Part model, mm, in its own coordinate system. A direction names the side the tool comes from. Coordinates: 2 decimals unless noted, no trailing zeros. Loops run counter-clockwise (first coordinate to the right, second up) from the corner with the lowest first, then second, coordinate; pieces in that order, holes last. Notation, with made-up numbers: M 54,9.5 L 93,9.5 A31 cw 93,44.5 Z; hole C -23,56 d6. An arc over 180 degrees is marked long. Use CSV: the item, a comma, the result in double quotes. Start each with the question number.
from build123d import *

# Parameters (mm, degrees)
F0_R     = 3.175
F1_DEPTH = 25.4
F2_R     = 12.7
F3_R     = 12.69999


# Not quite as in the source:
# - a fillet or chamfer is up to 0.001 mm smaller than in the source, because OpenCascade refuses the exact size


with BuildPart() as f1:
    # F0 (on Front) → F1 (new body)
    with BuildSketch(Plane.XZ):
        with BuildLine():
            Line((0, 44.897188701), (0, -74.9478926185))
            Line((0, -74.9478926185), (25.4, -74.9478926185))
            Line((25.4, -74.9478926185), (25.4, 44.897188701))
            ThreePointArc((25.4, 44.897188701), (-28.9774724535, 99.2746611545), (-83.3549449071, 44.897188701))
            Line((-83.3549449071, 44.897188701), (-57.9549449071, 44.897188701))
            ThreePointArc((-57.9549449071, 44.897188701), (-28.9774724535, 73.8746611545), (0, 44.897188701))
        make_face()
        with Locations((12.7, -62.2478926185)):
            Circle(F0_R, mode=Mode.SUBTRACT)
    extrude(amount=F1_DEPTH)

    # F2
    f2_edges = [f1.edges().sort_by_distance(p)[0] for p in [
        (-70.654945, -25.4, 44.897189),
    ]]
    fillet(f2_edges, radius=F2_R)

    # F3 (radius 12.7 in the source; OpenCascade refuses exactly that, so slightly less here)
    f3_edges = [f1.edges().sort_by_distance(p)[0] for p in [
        (-70.654945, 0, 44.897189),
    ]]
    fillet(f3_edges, radius=F3_R)


solid = f1.part
1. Wall check: probe 1 along X at (y, z) = (-9, 15); probe 2 along Z at (x, y) = (15, -2); probe 3 along Z at (x, y) = (12.7, -15.25). Give the ranges that are in metal, low to high.
2. Pin check, flat tips, straight feed: pin 1 (8 mm diameter, centred on x = -21.5, y = -7.5, fed in from +Z); pin 2 (12 mm diameter, centred on y = -9, z = -38.5, fed in from -X); pin 3 (3 mm diameter, centred on x = -39, y = -21.5, fed in from +Z). Stop position of each tip, or through.
3. Slice it at D-D, the plane z = -22. List the corners of the cut face in (x, y), and give its area (3 significant figures).
4. Slice it at A-A, the plane z = 51. List the corners of the cut face in (x, y).
5. Tool access for faces 5 (the face through (-68.99, -3.82, 48.52)), 6 (the face through (12.012, -12.522, -65.347)), 7 (the face through (-68.99, -21.58, 48.52)): list every direction of +Z, -Z, +X, -X, +Y, -Y with a clear straight run to the whole face (end or side of a thin tool).
6. Slice it at C-C, the plane y = -7.25. List the corners of the cut face in (x, z) (3 decimals), and give its area (3 significant figures).
7. Two-plate mould, pull along X, no slides. Class faces 1 (the face through (25.4, -13, -16)), 2 (the face through (3, -25.4, 38)), 3 (the face through (-29.615, -12.522, 73.868)), 4 (the face through (0, -13, -14)): pulls with the +X half, pulls with the -X half, needs draft (parallel to the pull), parting line crosses it, or undercut.
8. Slice it at B-B, the plane x = 12.7. List the corners of the cut face in (y, z).
Found:
1,probe 1,"0 to 25.4"
1,probe 2,"-74.95 to -64.44, -60.06 to 76.88"
1,probe 3,"-74.95 to -65.42, -59.07 to 79.82"
2,pin 1,"z = 99.16"
2,pin 2,"x = 0"
2,pin 3,"z = 98.6"
3,outline,"M 0,-25.4 L 25.4,-25.4 L 25.4,0 L 0,0 Z"
3,area,"645 mm^2"
4,outline,"M -83.01,-23.55 L -57.31,-23.55 L -57.31,-1.85 L -83.01,-1.85 Z; M -0.65,-25.4 L 25.06,-25.4 L 25.06,0 L -0.65,0 Z"
5,face 5,"-Z, -X, +Y"
5,face 6,"+Y, -Y"
5,face 7,"-Z, -X, -Y"
6,outline,"M -83.341,46.126 L -57.929,46.126 A28.977 cw 0,44.897 L 0,-74.948 L 25.4,-74.948 L 25.4,44.897 A54.377 ccw Z; hole C 12.7,-62.248 d6.35"
6,area,"6,310 mm^2"
7,face 1,"pulls with the +X half"
7,face 2,"needs draft"
7,face 3,"undercut"
7,face 4,"pulls with the -X half"
8,outline,"M -25.4,-74.95 L 0,-74.95 L 0,-65.42 L -25.4,-65.42 Z; M -25.4,-59.07 L 0,-59.07 L 0,79.82 L -25.4,79.82 Z"
